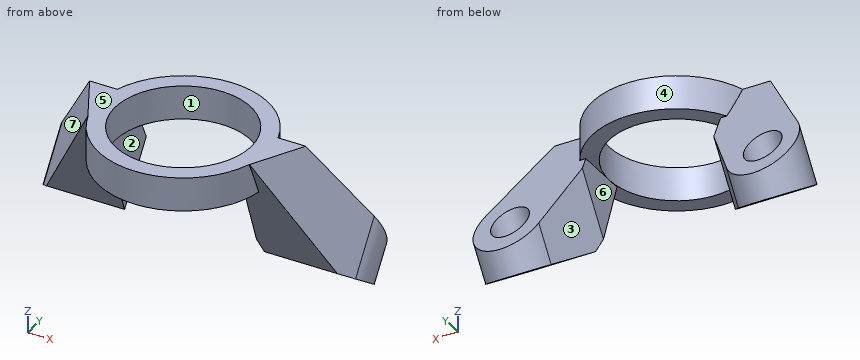
from build123d import *

# Parameters (mm, degrees)
SKETCH_R             = 10
PAD_DEPTH            = 4
PAD001_DEPTH         = 19.225
PAD001_DEPTH_BACK    = 19.225
SKETCH002_W          = 16
SKETCH002_H          = 14.708531
POCKET_DEPTH         = 100
POCKET_DEPTH_BACK    = 100
SKETCH005_R          = 2.225
POCKET002_DEPTH      = 100
POCKET002_DEPTH_BACK = 100
SKETCH006_R          = 8
POCKET003_DEPTH      = 18.2946687632


with BuildPart() as part:
    # Sketch → Pad (new body)
    with BuildSketch(Plane.XY):
        Circle(SKETCH_R)
    extrude(amount=PAD_DEPTH)

    # Sketch001 → Pad001 (join, two sides)
    with BuildSketch(Plane.YZ) as pad001_sk:
        Polygon((-3, 4), (3, 4), (10.4649812857, -11.8362126303), (8.7442519767, -14.2936687632), (1.8224172024, -9.446947876), align=None)
    extrude(amount=PAD001_DEPTH)
    extrude(pad001_sk.sketch, amount=-PAD001_DEPTH_BACK)

    # Sketch002 → Pocket (cut, two sides)
    with BuildSketch(Plane.XZ) as pocket_sk:
        with Locations((0, -7.3542655)):
            Rectangle(SKETCH002_W, SKETCH002_H)
    extrude(amount=-POCKET_DEPTH, mode=Mode.SUBTRACT)
    extrude(pocket_sk.sketch, amount=POCKET_DEPTH_BACK, mode=Mode.SUBTRACT)

    # Sketch005 (on Face5 of Pocket) → Pocket002 (cut, two sides)
    with BuildSketch(Plane(origin=(0, -3.8390566992, -5.4827411727), x_dir=(1, 0, 0), z_dir=(0, -0.5735764364, -0.8191520443))) as pocket002_sk:
        with Locations((-15, -11.136383474)):
            Circle(SKETCH005_R)
        with Locations((15, -11.136383474)):
            Circle(SKETCH005_R)
        with BuildLine():
            ThreePointArc((-18.5274170715, -8.8108827099), (-17.1496679718, -14.7736286694), (-11.2616841653, -13.1050428452))
            Line((-11.2616841653, -13.1050428452), (-8, -6.911383474))
            Line((-8, -6.911383474), (-8, -15.402658))
            Line((-8, -15.402658), (8, -15.402658))
            Line((8, -15.402658), (8, -5.4984980053))
            Line((11.1141301433, -12.7948889631), (8, -5.4984980053))
            ThreePointArc((11.1141301433, -12.7948889631), (17.0000496384, -14.8579995805), (18.5274170715, -8.8108827099))
            Line((9.4653449469, 4.9348482776), (18.5274170715, -8.8108827099))
            Line((9.4653449469, 4.9348482776), (21.017342039, 4.9348482776))
            Line((21.017342039, -22.489232832), (21.017342039, 4.9348482776))
            Line((-21.017342039, -22.489232832), (21.017342039, -22.489232832))
            Line((-21.017342039, 4.9348482776), (-21.017342039, -22.489232832))
            Line((-21.017342039, 4.9348482776), (-9.4653449469, 4.9348482776))
            Line((-9.4653449469, 4.9348482776), (-18.5274170715, -8.8108827099))
        make_face()
    extrude(amount=-POCKET002_DEPTH, mode=Mode.SUBTRACT)
    extrude(pocket002_sk.sketch, amount=POCKET002_DEPTH_BACK, mode=Mode.SUBTRACT)

    # Sketch006 (on Face23 of Pocket002) → Pocket003 (cut, through all)
    with BuildSketch(Plane.XY.offset(4)):
        Circle(SKETCH006_R)
    extrude(amount=-POCKET003_DEPTH, mode=Mode.SUBTRACT)


solid = part.part
For this review, take the finished solid that the model builds, in its own axes (mm). Face numbers are marked on the shaded views. A direction names the side the tool comes from. Round coordinates to 2 decimals unless told otherwise and drop trailing zeros. Loops run counter-clockwise (first coordinate to the right, second up) from the corner with the lowest first, then second, coordinate; pieces in that order, holes last. Notation, with made-up numbers: (-8, 28) - (51, 28) arc R18 ccw to (51, 57) - close; hole circle Ø3 at (7.5, -35.75). An arc over 180 degrees is marked (long way). Put each result on its own line as item: value. Start each with the question number.
1. For probe 1 along Y at (x, z) = (0, 2.55); probe 2 along X at (y, z) = (7.25, -9); probe 3 along Z at (x, y) = (-7, 6.75), list the stretches that pass through material, from the lowest coordinate up. Write a range as [from, to].
2. Consider section C-C on x = 15.5. State the section outline as (y, z) points.
3. Consider section B-B on z = -0.75. State the section outline as (x, y) points, plus the area to 3 significant figures.
4. For the marked faces 1, 2 and 3, list the 3-axis set-ups (+Z, -Z, +X, -X, +Y, -Y) from which the entire face can be reached by the end or side of a thin tool; tool diameter is ignored.
5. Consider section A-A on x = 0. State the section outline as (y, z) points, plus the area to 3 significant figures.
6. Mouldability with a two-part tool opening along X and no side actions: class the marked faces 4, 5, 6 and 7 as +X half, -X half, draft (parallel to the pull), parting line (faces both ways), or undercut.
7. Consider section D-D on z = -4.25. State the section outline as (x, y) points, plus the area to 3 significant figures.
8. Insertion check: P1, Ø6.5, axis at y = 2.5, z = -2.5, coming from the +X side; P2, Ø6, axis at y = 3.5, z = -10, coming from the +X side (3 decimals); P3, Ø5, axis at x = -14, y = -3.5, coming from the -Z side; P4, Ø8, axis at y = 0.5, z = -0.5, coming from the -X side. Each pin has a flat end and moves straight along its axis. Give the tip position at first contact, or say it passes through.
Result sheet:
1. probe 1: [-10, -8], [8, 10]
1. probe 2: [-19.22, -17.22], [-12.78, -10.21], [10.39, 12.78], [17.22, 19.22]
1. probe 3: [0, 4]
2. outline: (0.71, -6.34) - (1.82, -9.45) - (3.51, -10.63) - (7.32, -5.17) - (4.99, -0.23) - close; (7.06, -13.11) - (8.72, -14.28) - (10.45, -11.81) - (9.45, -9.69) - close
3. outline: (-15.83, 5.24) - (-12.3, -1.3) - (-8, -1.3) - (-8, 5.24) - close; (8, -1.3) - (12.3, -1.3) - (15.83, 5.24) - (8, 5.24) - close
3. area: 79.3 mm^2
4. face 1: +Z, -Z
4. face 2: -Z, +Y, -Y
4. face 3: -Z, +Y
5. outline: (-10, 0) - (-8, 0) - (-8, 4) - (-10, 4) - close; (8, 0) - (10, 0) - (10, 4) - (8, 4) - close
5. area: 16.0 mm^2
6. face 4: parting line
6. face 5: draft
6. face 6: undercut
6. face 7: -X half
7. outline: (-18.05, 6.89) - (-14.3, -0.04) - (-8, -0.04) - (-8, 5.46) - (-8.62, 6.89) - close; (8, -0.04) - (14.3, -0.04) - (18.05, 6.89) - (9.1, 6.89) - (8, 3.74) - close
7. area: 111 mm^2
8. P1: x = 17.16
8. P2: x = 19.225
8. P3: through
8. P4: x = -15.81
